Autodesk Inventor part; units mm, degrees
ref_plane "YZ Plane" through (0, 0, 0) normal (1, 0, 0) x (0, 1, 0)
ref_plane "XZ Plane" through (0, 0, 0) normal (0, 1, 0) x (-1, 0, 0)
ref_plane "XY Plane" through (0, 0, 0) normal (0, 0, 1) x (1, 0, 0)
sketch "Sketch1" plane through (0, 0, 0) normal (0, 1, 0) x (-1, 0, 0)
  line L0 (-35, 27) -> (35, 27)
  line L1 (35, 27) -> (35, -27)
  line L2 (35, -27) -> (-35, -27)
  line L3 (-35, -27) -> (-35, 27)
  line L4 (-35, 27) -> (35, -27) construction
  line L5 (35, 27) -> (-35, -27) construction
  line L6 (30, 21.5) -> (-30, 21.5) construction
  line L7 (-30, 21.5) -> (-30, -21.5) construction
  line L8 (-30, -21.5) -> (30, -21.5) construction
  line L9 (30, -21.5) -> (30, 21.5) construction
  line L10 (30, 21.5) -> (-30, -21.5) construction
  line L11 (-30, 21.5) -> (30, -21.5) construction
  circle A0 centre (30, 21.5) radius 1.5
  circle A1 centre (30, -21.5) radius 1.5
  circle A2 centre (-30, -21.5) radius 1.5
  circle A3 centre (-30, 21.5) radius 1.5
  point P0 (0, 0)
  dimension "d0" = 70
  dimension "d1" = 54
  dimension "d2" = 43
  dimension "d3" = 60
  dimension "d4" = 3
  dimension "d5" = 3
  dimension "d6" = 3
  dimension "d7" = 3
extrude "Extrusion1" add sketch "Sketch1" along normal blind 2
fillet "Fillet1" radius 2 4 edges at (35, 1, 27) (35, 1, -27) (-35, 1, 27) (-35, 1, -27)
sketch "Sketch2" plane through (0, 0, 0) normal (0, -1, 0) x (1, 0, 0)
  circle A0 centre (0, 0) radius 3.5
  dimension "d11" = 7
extrude "Extrusion2" cut sketch "Sketch2" against normal blind 1
sketch "Sketch3" plane through (0, 0, 0) normal (0, -1, 0) x (1, 0, 0)
  line L0 (-33, 27) -> (33, 27)
  circle A0 centre (0, 0) radius 3.5
  line L1 (0, 27) -> (0, 0)
  line L2 (0.5, 27) -> (-0.5, 27)
  line L3 (-0.5, 27) -> (-0.5, 0)
  line L4 (-0.5, 0) -> (0.5, 0)
  line L5 (0.5, 0) -> (0.5, 27)
  point P0 (-0.5, 27)
  dimension "d14" = 0.5
  dimension "d15" = 0.5
extrude "Extrusion3" cut sketch "Sketch3" against normal blind 1 contours L0 L1 A0 L3 | L0 L5 A0 L1 | A0 L1 L4 L3 | A0 L5 L4 L1
chamfer "Chamfer1" distance 1.4 angle 45 4 edges at (-28.5, 2, -21.5) (-28.5, 2, 21.5) (31.5, 2, 21.5) (31.5, 2, -21.5)
properties part number "Bed"
Build history of the part. All positions in model axes, mm. A direction names the side the tool comes from. Coordinates: 2 decimals unless noted, no trailing zeros. Write each loop counter-clockwise with the first axis right and the second up, starting at its lowest first coordinate (ties: lowest second). Pieces come first, ordered by that corner, then holes.
1. Pull direction Z, two halves, no side cores. Call faces 3 (the cylindrical face through (31.11, 0.3, -22.51)), 4 (the flat face through (0.5, 1.2, 27)), 5 (the flat face through (35, 1, 0)), 6 (the flat face through (0, 1, -27)): released by +Z, released by -Z, zero draft, split by the parting line, or undercut.
Answer block:
face 3: undercut
face 4: released by +Z
face 5: zero draft
face 6: released by -Z
2. Drill centre lines: probe 1 along Z at (x, y) = (30, 0.25); probe 2 along X at (y, z) = (0.75, 0); probe 3 along Z at (x, y) = (31, 0.1). Where is each one in solid material? Low to high.
Answer block:
probe 1: z = -27 to -23, -20 to 20, 23 to 27
probe 2: x = -35 to -3.5, 3.5 to 35
probe 3: z = -27 to -22.62, -20.38 to 20.38, 22.62 to 27
3. Band-saw the part on A-A, the plane z = 21.5. Give the cut face in (x, y), and give its area (3 significant figures).
Answer block:
outline: (-35, 0) - (-31.5, 0) - (-31.5, 0.6) - (-32.9, 2) - (-35, 2) - close; (-28.5, 0) - (-0.5, 0) - (-0.5, 1) - (0.5, 1) - (0.5, 0) - (28.5, 0) - (28.5, 0.6) - (27.1, 2) - (-27.1, 2) - (-28.5, 0.6) - close; (31.5, 0) - (35, 0) - (35, 2) - (32.9, 2) - (31.5, 0.6) - close
area: 123 mm2
4. Band-saw the part on C-C, the plane z = 1.5. Give the cut face in (x, y).
Answer block:
outline: (-35, 0) - (-3.16, 0) - (-3.16, 1) - (3.16, 1) - (3.16, 0) - (35, 0) - (35, 2) - (-35, 2) - close
5. 3-axis set-ups, long thin cutter, end or side, ignore diameter. For faces 1 (the cylindrical face through (-34.43, 1.01, 26.4)), 2 (the cylindrical face through (-0.1, 0.5, -3.5)): which of +Z, -Z, +X, -X, +Y, -Y reach the whole face in a straight line?
Answer block:
face 1: +Z, -X, +Y, -Y
face 2: -Y
6. Drop a flat-ended pin along its axis: pin 1 (7.5 mm diameter, centred on x = -1, z = 19, fed in from -Y). Give the stop position or say it passes through.
Answer block:
pin 1: stops at y = 0
7. Band-saw the part on B-B, the plane x = -30. Give the cut face in (y, z), and give its area (3 significant figures).
Answer block:
outline: (0, -27) - (2, -27) - (2, -24.4) - (0.6, -23) - (0, -23) - close; (0, -20) - (0.6, -20) - (2, -18.6) - (2, 18.6) - (0.6, 20) - (0, 20) - close; (0, 23) - (0.6, 23) - (2, 24.4) - (2, 27) - (0, 27) - close
area: 92.1 mm2
